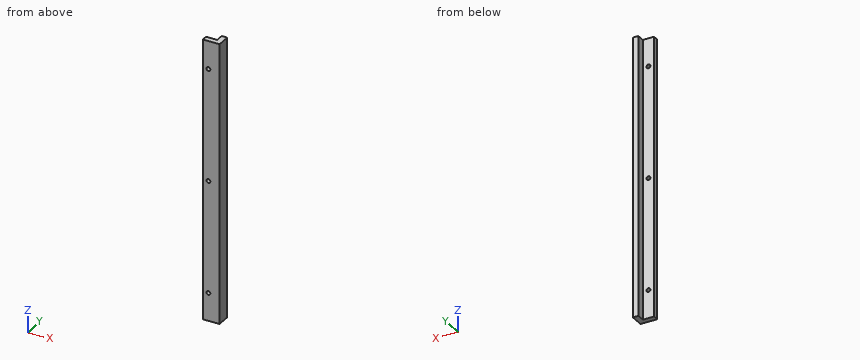
from build123d import *

# Parameters (mm, degrees)
SKETCH_1_W          = 15
SKETCH_1_H          = 250
EXTRUDE_1_DEPTH     = 5
SKETCH_2_W          = 250
SKETCH_2_H          = 12
EXTRUDE_2_DEPTH     = 5
SKETCH_3_R          = 1.75
CUT_EXTRUDE_1_DEPTH = 5


with BuildPart() as part:
    # 草图1 → 凸台-拉伸1 (new body)
    with BuildSketch(Plane(origin=(0, 0, 0), x_dir=(1, 0, 0), z_dir=(0, 1, 0))):
        Rectangle(SKETCH_1_W, SKETCH_1_H)
    extrude(amount=EXTRUDE_1_DEPTH)

    # 草图2 → 凸台-拉伸2 (add)
    with BuildSketch(Plane(origin=(7.5, 0, 0), x_dir=(0, 0, -1), z_dir=(1, 0, 0))):
        with Locations((0, 6)):
            Rectangle(SKETCH_2_W, SKETCH_2_H)
    extrude(amount=-EXTRUDE_2_DEPTH)

    # 草图3 → 切除-拉伸1 (cut)
    with BuildSketch(Plane(origin=(0, 5, 0), x_dir=(1, 0, 0), z_dir=(0, 1, 0))):
        with Locations(Location((-2.5, 100, 0), (0, 0, 270))):
            Circle(SKETCH_3_R)
        with Locations(Location((-2.5, 0, 0), (0, 0, 270))):
            Circle(SKETCH_3_R)
        with Locations(Location((-2.5, -100, 0), (0, 0, 270))):
            Circle(SKETCH_3_R)
    extrude(amount=-CUT_EXTRUDE_1_DEPTH, mode=Mode.SUBTRACT)


solid = part.part
Geometry: final body of the model. Coordinates: model frame, mm. Coordinates: 2 decimals unless noted, no trailing zeros. Loops run counter-clockwise (first coordinate to the right, second up) from the corner with the lowest first, then second, coordinate; pieces in that order, holes last. Notation, with made-up numbers: M 12.25,46.5 L 34.25,46.5 A14 ccw 34.25,62.5 Z; hole C 88.25,47 d4. An arc over 180 degrees is marked long. One line per item, written item: value. Start each with the question number.
1) Material intervals for L1, parallel to X at y = 2.05, z = -100; L2, parallel to Z at x = -4, y = 3.5; L3, parallel to Y at x = 0.5, z = 14, sorted ascending. Write a range as from..to.
2) Cut plane B-B (y = 9.5). Return loops of the section in (x, z), then the cut area to 3 significant figures.
3) Pin query (flat end, axial travel): P1, Ø5.5, axis at y = 10, z = -31, coming from the -X side; P2, Ø4, axis at x = 4.5, z = 43, coming from the -Y side; P3, Ø5, axis at x = -3, z = 4.5, coming from the +Y side. Return the tip coordinate at first contact, or that it passes through.
4) Cut plane A-A (z = 11.5). Return loops of the section in (x, y).
Evaluation:
1. L1: -7.5..-4.25, -0.75..7.5
1. L2: -125..-100.9, -99.1..-0.9, 0.9..99.1, 100.9..125
1. L3: 0..5
2. outline: M 2.5,-125 L 7.5,-125 L 7.5,125 L 2.5,125 Z
2. area: 1,250 mm^2
3. P1: x = 2.5
3. P2: y = 0
3. P3: y = 5
4. outline: M -7.5,0 L 7.5,0 L 7.5,12 L 2.5,12 L 2.5,5 L -7.5,5 Z
